Could you check a few things on this model? Use its own coordinates, in mm. A direction names the side the tool comes from. Give positions to 0.01 mm unless a question says otherwise; leave off trailing zeros. Loops run counter-clockwise (first coordinate to the right, second up) from the corner with the lowest first, then second, coordinate; pieces in that order, holes last.
1. I need wall thicknesses on line 1 along Y through (x, z) = (45, -0.6); line 2 along Z through (x, y) = (44, -9). Which ranges of each line are inside material? Lowest first, please.
2. Imagine slicing it at D-D (x = 18). List the corners of the cut face in (y, z) for me, plus the area to 3 significant figures.
3. Thinking about a two-plate mould opening in Y: for faces 1 (the flat face through (24, 0, 0.75)), 2 (the flat face through (0, 15, 0)), 3 (the cylindrical face through (38.03, 5.3, 0.01)), 4 (the cylindrical face through (44.34, -4.324, 0.01)), which applies, +Y half, -Y half, draft (parallel to the pull), parting line (faces both ways), or undercut?
4. For P1, Ø1, axis at x = 45.5, y = 3, coming from the -Z side; P2, Ø3, axis at x = 25.08, y = -5, coming from the +Z side, each with a flat end and sliding along its axis, tell me the tip position at first contact or that it passes through.
5. Imagine slicing it at C-C (y = 9.25). List the corners of the cut face in (x, z) for me.
6. Imagine slicing it at A-A (z = 0). Count the separate pieces of the cut face and the enclosed holes in it, plus the area to 3 significant figures.
7. For faces 5 (the cylindrical face through (34.03, -4.7, 0.01)), 6 (the flat face through (34, 10, 0)), 7 (the flat face through (34, -10, 0)), which set-ups out of +Z, -Z, +X, -X, +Y, -Y let a thin tool reach every point of the face, with its end or its side?
```python
from build123d import *

# Parameters (mm, degrees)
BOSS_EXTRUDE1_DEPTH      = 15
BOSS_EXTRUDE1_DEPTH_BACK = 15
SKETCH2_R                = 1
CUT_EXTRUDE1_DEPTH       = 62.064988474
FILLET1_R                = 30
FILLET2_R                = 10


with BuildPart() as part:
    # Sketch1 → Boss-Extrude1 (new, two sides: drawn at the far end of the back side and taken through both)
    with BuildSketch(Plane(origin=(0, 0, 0), x_dir=(1, 0, 0), z_dir=(0, 1, 0)).offset(-BOSS_EXTRUDE1_DEPTH_BACK)):
        with BuildLine():
            Line((1.5612495, 0.75), (59.1512495, 0.75))
            Line((59.1512495, 0.75), (59.1512495, -0.75))
            Line((59.1512495, -0.75), (1.5612495, -0.75))
            ThreePointArc((1.5612495, -0.75), (1.344743149, -0.799306091), (1.170937125, -0.9375))
            ThreePointArc((1.170937125, -0.9375), (-1.5, 0), (1.170937125, 0.9375))
            ThreePointArc((1.170937125, 0.9375), (1.344743149, 0.799306091), (1.5612495, 0.75))
        make_face()
    extrude(amount=BOSS_EXTRUDE1_DEPTH + BOSS_EXTRUDE1_DEPTH_BACK)

    # Sketch2 → Cut-Extrude1 (cut, through all)
    with BuildSketch(Plane.XY.offset(0.75)):
        with Locations((49.0772495, 5)):
            Circle(SKETCH2_R)
        with Locations((45.0772495, 5)):
            Circle(SKETCH2_R)
        with Locations((41.0772495, 5)):
            Circle(SKETCH2_R)
        with Locations((37.0772495, 5)):
            Circle(SKETCH2_R)
        with Locations((33.0772495, 5)):
            Circle(SKETCH2_R)
        with Locations((29.0772495, 5)):
            Circle(SKETCH2_R)
        with Locations((25.0772495, 5)):
            Circle(SKETCH2_R)
        with Locations((21.0772495, 5)):
            Circle(SKETCH2_R)
        with Locations((45.0772495, -5)):
            Circle(SKETCH2_R)
        with Locations((41.0772495, -5)):
            Circle(SKETCH2_R)
        with Locations((37.0772495, -5)):
            Circle(SKETCH2_R)
        with Locations((33.0772495, -5)):
            Circle(SKETCH2_R)
        with Locations((29.0772495, -5)):
            Circle(SKETCH2_R)
        with Locations((25.0772495, -5)):
            Circle(SKETCH2_R)
        with Locations((21.0772495, -5)):
            Circle(SKETCH2_R)
        with Locations((49.0772495, -5)):
            Circle(SKETCH2_R)
        Polygon((49.0772495, 10), (21.0772495, 10), (2.0652495, 15), (59.1512495, 15), (59.1512495, 5), align=None)
        Polygon((49.0772495, -10), (21.0772495, -10), (2.0652495, -15), (59.1512495, -15), (59.1512495, -5), align=None)
    extrude(amount=-CUT_EXTRUDE1_DEPTH, mode=Mode.SUBTRACT)

    # Fillet1
    fillet1_edges = [part.edges().sort_by_distance(p)[0] for p in [
        (49.0772495, 10, 0),
        (21.0772495, 10, 0),
        (49.0772495, -10, 0),
        (21.0772495, -10, 0),
    ]]
    fillet(fillet1_edges, radius=FILLET1_R)

    # Fillet2
    # the kernel refuses this fillet: 10 mm, written as the material it takes off along each edge
    with BuildSketch(Plane(origin=(59.1512495, -5, 18.566207641), x_dir=(-0.9044112472912746, -0.42666180491466615, 0), z_dir=(0, 0, -1))) as fillet2_piece_1:
        with BuildLine():
            CenterArc((6.353468821, 9.970077682), FILLET2_R, 205.255895662, 69.177572528)
            Line((-2.690643652, 5.703459633), (-3.595054899, 5.276797828))
            Line((-3.595054899, 5.276797828), (-0.904411247, -0.426661805))
            Line((-0.904411247, -0.426661805), (-0.019905188, -0.999801872))
            ThreePointArc((-0.019905188, -0.999801872), (4.190379521, -1.083624989), (7.20378448, -0.997007768))
            Line((7.20378448, -0.997007768), (7.126483056, 0))
        make_face()
    extrude(amount=37.132415281, mode=Mode.SUBTRACT)
    with BuildSketch(Plane(origin=(59.1512495, 5, 18.566207641), x_dir=(0, -1, 0), z_dir=(0, 0, -1))) as fillet2_piece_2:
        with BuildLine():
            CenterArc((6.306267918, 10), FILLET2_R, 200.822427472, 69.177572528)
            Line((-3.040598123, 6.44527143), (-3.975284728, 6.089798573))
            ThreePointArc((-3.975284728, 6.089798573), (-2.767917517, 3.327484976), (-0.895739275, -0.444579747))
            Line((-0.895739275, -0.444579747), (0, -1))
            Line((0, -1), (6.306267918, -1))
            Line((6.306267918, -1), (6.306267918, 0))
        make_face()
    extrude(amount=37.132415281, mode=Mode.SUBTRACT)


solid = part.part
```
Derived:
1. line 1: y = -9.85 to -6, -4 to 4, 6 to 9.85
1. line 2: z = -0.75 to 0.75
2. outline: (-10.82, -0.75) - (10.82, -0.75) - (10.82, 0.75) - (-10.82, 0.75) - close
2. area: 32.5 mm2
3. face 1: draft
3. face 2: +Y half
3. face 3: undercut
3. face 4: undercut
4. P1: stops at z = -0.75
4. P2: stops at z = 0.75
5. outline: (1.17, -0.94) arc R0.5 cw to (1.56, -0.75) - (48.71, -0.75) - (48.71, 0.75) - (1.56, 0.75) arc R0.5 cw to (1.17, 0.94) arc R1.5 ccw (long way) to start
6. separate pieces: 1
6. enclosed holes: 16
6. area: 1,220 mm2
7. face 5: +Z, -Z
7. face 6: +Z, -Z, +X, +Y
7. face 7: +Z, -Z, +X, -Y
